Print and shaded views of the part. All mm, measured from the part's lowest x, y and z. Give positions to 0.01 mm unless a question says otherwise; leave off trailing zeros. Loops run counter-clockwise (first coordinate to the right, second up) from the corner with the lowest first, then second, coordinate; pieces in that order, holes last.
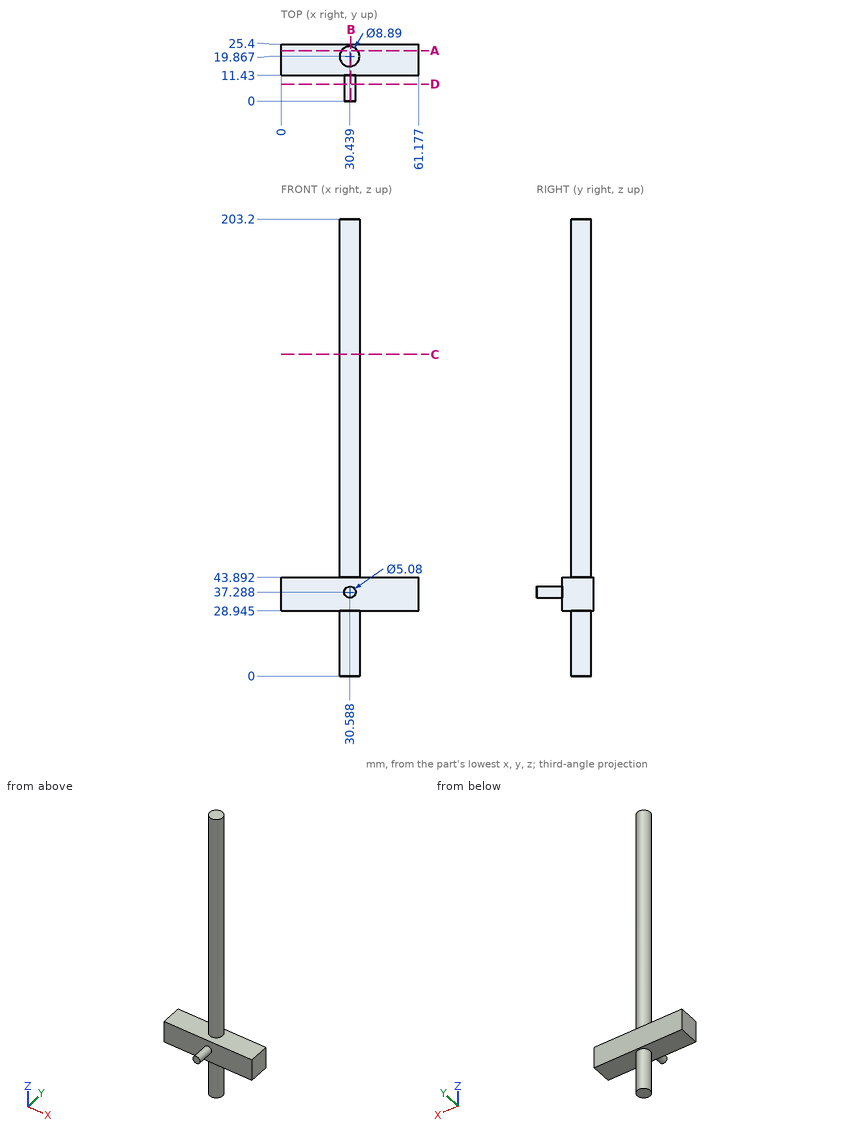
1. Saw through at D-D, the plane y = 7.5. List the corners of the cut face in (x, z), and give its area (3 significant figures).
Responses:
outline: circle Ø5.08 at (30.59, 37.29)
area: 20.3 mm2
2. Saw through at A-A, the plane y = 22.5. List the corners of the cut face in (x, z) (1 decimal), and give its area (3 significant figures).
Responses:
outline: (0, 28.9) - (26.9, 28.9) - (26.9, 0) - (34, 0) - (34, 28.9) - (61.2, 28.9) - (61.2, 43.9) - (34, 43.9) - (34, 203.2) - (26.9, 203.2) - (26.9, 43.9) - (0, 43.9) - close
area: 2,260 mm2
3. Probe line 1 along Z through (x, y) = (21.5, 16.5) (1 decimal); line 2 along Y through (x, z) = (34, 34.5); line 3 along X through (y, z) = (17.75, 119.5). List the from-to ranges inside material, lowest first.
Responses:
line 1: z = 28.9 to 43.9
line 2: y = 11.43 to 25.4
line 3: x = 26.53 to 34.35
4. Drop flat-ended pins along their axis: pin 1 (6 mm diameter, centred on x = 13, z = 45.5, fed in from -Y); pin 2 (4 mm diameter, centred on x = 19, y = 18, fed in from +Z); pin 3 (8 mm diameter, centred on x = 28.5, z = 95.5, fed in from -Y). Give the stop position or say it passes through.
Responses:
pin 1: stops at y = 11.43
pin 2: stops at z = 43.89
pin 3: stops at y = 15.42
5. Saw through at C-C, the plane z = 143. List the corners of the cut face in (x, y) (1 decimal).
Responses:
outline: circle Ø8.9 at (30.4, 19.9)
6. Saw through at B-B, the plane x = 31. List the corners of the cut face in (y, z) (1 decimal), and give its area (3 significant figures).
Responses:
outline: (0, 34.8) - (11.4, 34.8) - (11.4, 28.9) - (15.5, 28.9) - (15.5, 0) - (24.3, 0) - (24.3, 28.9) - (25.4, 28.9) - (25.4, 43.9) - (24.3, 43.9) - (24.3, 203.2) - (15.5, 203.2) - (15.5, 43.9) - (11.4, 43.9) - (11.4, 39.8) - (0, 39.8) - close
area: 1,930 mm2
